```python
from build123d import *

# Parameters (mm, degrees)
SKETCH1_W                  = 52
SKETCH1_H                  = 18
BOSS_EXTRUDE1_DEPTH        = 3
SKETCH2_W                  = 32
SKETCH2_H                  = 14
CUT_EXTRUDE1_DEPTH         = 2.65
FILLET1_SIZE               = 4.2
F_2_6_2_6_DIAMETER_HOLE1_D = 2.6


with BuildPart() as part:
    # Sketch1 → Boss-Extrude1 (new body)
    with BuildSketch(Plane(origin=(0, 0, 0), x_dir=(1, 0, 0), z_dir=(0, 1, 0))):
        Rectangle(SKETCH1_W, SKETCH1_H)
    extrude(amount=BOSS_EXTRUDE1_DEPTH)

    # Sketch2 → Cut-Extrude1 (cut)
    with BuildSketch(Plane(origin=(0, 3, 0), x_dir=(1, 0, 0), z_dir=(0, 1, 0))):
        Rectangle(SKETCH2_W, SKETCH2_H)
    extrude(amount=-CUT_EXTRUDE1_DEPTH, mode=Mode.SUBTRACT)

    # Fillet1
    # a fillet whose section is not a circle: 4.2 mm, written as the material it adds along each edge
    with BuildSketch(Plane(origin=(16, 3, 7), x_dir=(0, 0, -1), z_dir=(0, -1, 0)), Plane(origin=(-16, 3, 7), x_dir=(1, 0, 0), z_dir=(0, -1, 0)), Plane(origin=(16, 3, -7), x_dir=(-1, 0, 0), z_dir=(0, -1, 0))) as fillet1_piece_1:
        with BuildLine():
            Bezier((FILLET1_SIZE, 0), (0, 0), (0, -FILLET1_SIZE), weights=[1, 1.857142857, 1])
            Line((0, -FILLET1_SIZE), (-FILLET1_SIZE * 0.02, -FILLET1_SIZE))
            Line((-FILLET1_SIZE * 0.02, -FILLET1_SIZE), (-FILLET1_SIZE * 0.02, FILLET1_SIZE * 0.02))
            Line((-FILLET1_SIZE * 0.02, FILLET1_SIZE * 0.02), (FILLET1_SIZE, FILLET1_SIZE * 0.02))
            Line((FILLET1_SIZE, FILLET1_SIZE * 0.02), (FILLET1_SIZE, 0))
        make_face()
    extrude(amount=2.65)
    with BuildSketch(Plane(origin=(-16, 3, -7), x_dir=(1, 0, 0), z_dir=(0, -1, 0))) as fillet1_piece_2:
        with BuildLine():
            Bezier((FILLET1_SIZE, 0), (0, 0), (0, FILLET1_SIZE), weights=[1, 1.857142857, 1])
            Line((0, FILLET1_SIZE), (-FILLET1_SIZE * 0.02, FILLET1_SIZE))
            Line((-FILLET1_SIZE * 0.02, FILLET1_SIZE), (-FILLET1_SIZE * 0.02, -FILLET1_SIZE * 0.02))
            Line((-FILLET1_SIZE * 0.02, -FILLET1_SIZE * 0.02), (FILLET1_SIZE, -FILLET1_SIZE * 0.02))
            Line((FILLET1_SIZE, -FILLET1_SIZE * 0.02), (FILLET1_SIZE, 0))
        make_face()
    extrude(amount=2.65)

    # Ø2.6 (2.6) Diameter Hole1 (through all)
    with Locations(Plane(origin=(0, 3, 0), x_dir=(1, 0, 0), z_dir=(0, 1, 0))):
        with Locations((-20.5, 6), (-20.5, -6), (20.5, 6), (20.5, -6)):
            Hole(F_2_6_2_6_DIAMETER_HOLE1_D / 2)


solid = part.part
```
CAD build for the part. Positions are in the model's coordinates, mm. A direction names the side the tool comes from. Give positions to 0.01 mm unless a question says otherwise; leave off trailing zeros. Write each loop counter-clockwise with the first axis right and the second up, starting at its lowest first coordinate (ties: lowest second). Pieces come first, ordered by that corner, then holes. Notation, with made-up numbers: M 89,66.25 L 133,66.25 A4 ccw 133,72.25 Z; hole C 85,-8.5 d1. An arc over 180 degrees is marked long. Return JSON: item names as keys, results as strings. Group by question number.
(1) Band-saw the part on C-C (z = 1.25). Give the cut face in (x, y).
(2) Mould opens along X. For faces 1 (the face through (26, 1, 0)), 2 (the face through (-26, 1, 0)), 3 (the face through (0, 2, -7)), 4 (the face through (0, 1, 9)) say: pulls with the +X half, pulls with the -X half, needs draft (parallel to the pull), parting line crosses it, or undercut.
(3) Flat gauge pins, fed straight in: pin 1 Ø10 at (x, z) = (-14, 1) entering from +Y; pin 2 Ø2 at (x, z) = (-20.5, 6) entering from +Y; pin 3 Ø5 at (x, z) = (-4.5, 0.5) entering from +Y. Where does each tip first touch, or does it go through?
(4) Band-saw the part on D-D (y = 1). State how many separate pieces and enclosed holes the cut face has, and give its area (3 significant figures).
(5) 3-axis set-ups, long thin cutter, end or side, ignore diameter. For faces 5 (the face through (0, 0.35, 0)), 6 (the face through (0, 3, -8)): which of +Z, -Z, +X, -X, +Y, -Y reach the whole face in a straight line?
(6) Band-saw the part on B-B (x = 10). Give the cut face in (y, z).
(7) Band-saw the part on A-A (x = 20.5). Give the cut face in (y, z).
(8) Drill centre lines: L1, parallel to Z at x = -20.5, y = 2.15; L2, parallel to Z at x = 12, y = 1.8; L3, parallel to X at y = 0.7, z = -6. Where is each one in solid material? Low to high. Write a range as [from, to].
Entries:
{
 "1": {"outline": "M -26,0 L 26,0 L 26,3 L 16,3 L 16,0.35 L -16,0.35 L -16,3 L -26,3 Z"},
 "2": {"face 1": "pulls with the +X half", "face 2": "pulls with the -X half", "face 3": "undercut", "face 4": "needs draft"},
 "3": {"pin 1": "stops at y = 3", "pin 2": "passes through", "pin 3": "stops at y = 0.35"},
 "4": {"separate pieces": "1", "enclosed holes": "5", "area": "473 mm^2"},
 "5": {"face 5": "+Y", "face 6": "+Z, -Z, +X, -X, +Y"},
 "6": {"outline": "M 0,-9 L 3,-9 L 3,-7 L 0.35,-7 L 0.35,7 L 3,7 L 3,9 L 0,9 Z"},
 "7": {"outline": "M 0,-9 L 3,-9 L 3,-7.3 L 0,-7.3 Z; M 0,-4.7 L 3,-4.7 L 3,4.7 L 0,4.7 Z; M 0,7.3 L 3,7.3 L 3,9 L 0,9 Z"},
 "8": {"L1": "z = [-9, -7.3], [-4.7, 4.7], [7.3, 9]", "L2": "z = [-9, -7], [7, 9]", "L3": "x = [-26, -21.8], [-19.2, -15.48], [15.48, 19.2], [21.8, 26]"}
}
